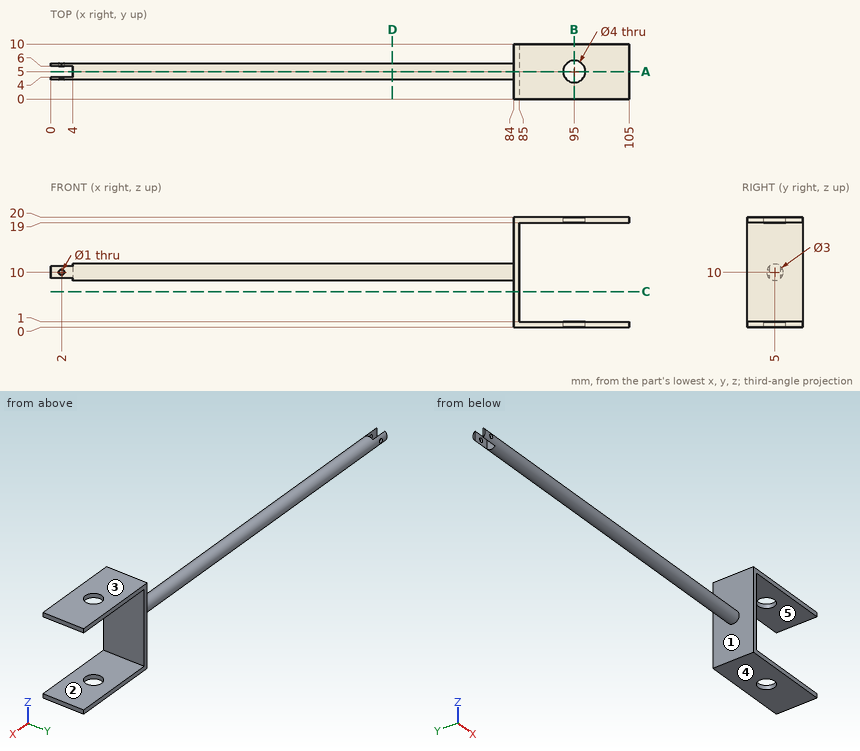
Verification items for this drawing (mm, ordinates from the low corner). A direction names the side the tool comes from. Give positions to 0.01 mm unless a question says otherwise; leave off trailing zeros. Write each loop counter-clockwise with the first axis right and the second up, starting at its lowest first coordinate (ties: lowest second). Pieces come first, ordered by that corner, then holes.
1) Thickness scan on line 1 (X direction, y = 5, z = 19.7); line 2 (Z direction, x = 99.5, y = 4); line 3 (X direction, y = 3, z = 9.5). Record the ranges inside material, lowest first.
Values follow:
line 1: x = 84 to 93, 97 to 105
line 2: z = 0 to 1, 19 to 20
line 3: x = 84 to 85
2) Cross-section at C-C (z = 6.5). Record the boundary of the cut face in (x, y), plus the area to 3 significant figures.
Values follow:
outline: (84, 0) - (85, 0) - (85, 10) - (84, 10) - close
area: 10.0 mm2
3) Go/stop test with flat-tipped pins: pin 1 Ø2.5 at (x, z) = (2, 9.5) entering from -Y; pin 2 Ø1 at (x, y) = (80.5, 6.5) entering from +Z; pin 3 Ø0.7 at (x, z) = (2.5, 10.5) entering from +Y. Record where each tip stops, or that it passes through.
Values follow:
pin 1: stops at y = 3.5
pin 2: stops at z = 11.12
pin 3: stops at y = 6.49
4) Release check for a two-part mould opening along Z. For the marked faces 1, 2 and 3 record: released by +Z, released by -Z, zero draft, split by the parting line, or undercut.
Values follow:
face 1: zero draft
face 2: undercut
face 3: released by +Z
5) Cross-section at B-B (x = 95). Record the boundary of the cut face in (y, z).
Values follow:
outline: (0, 0) - (3, 0) - (3, 1) - (0, 1) - close; (0, 19) - (3, 19) - (3, 20) - (0, 20) - close; (7, 0) - (10, 0) - (10, 1) - (7, 1) - close; (7, 19) - (10, 19) - (10, 20) - (7, 20) - close
6) Cross-section at A-A (y = 5). Record the boundary of the cut face in (x, z).
Values follow:
outline: (4, 8.5) - (84, 8.5) - (84, 0) - (93, 0) - (93, 1) - (85, 1) - (85, 19) - (93, 19) - (93, 20) - (84, 20) - (84, 11.5) - (4, 11.5) - close; (97, 0) - (105, 0) - (105, 1) - (97, 1) - close; (97, 19) - (105, 19) - (105, 20) - (97, 20) - close
7) Cross-section at D-D (x = 62). Record the boundary of the cut face in (y, z).
Values follow:
outline: circle Ø3 at (5, 10)
8) Set-up check for the marked faces 4 and 5: record each of +Z, -Z, +X, -X, +Y, -Y from which the full face is reachable in a straight line by a thin tool's end or side.
Values follow:
face 4: -Z, +X, -X, +Y, -Y
face 5: +X, +Y, -Y
